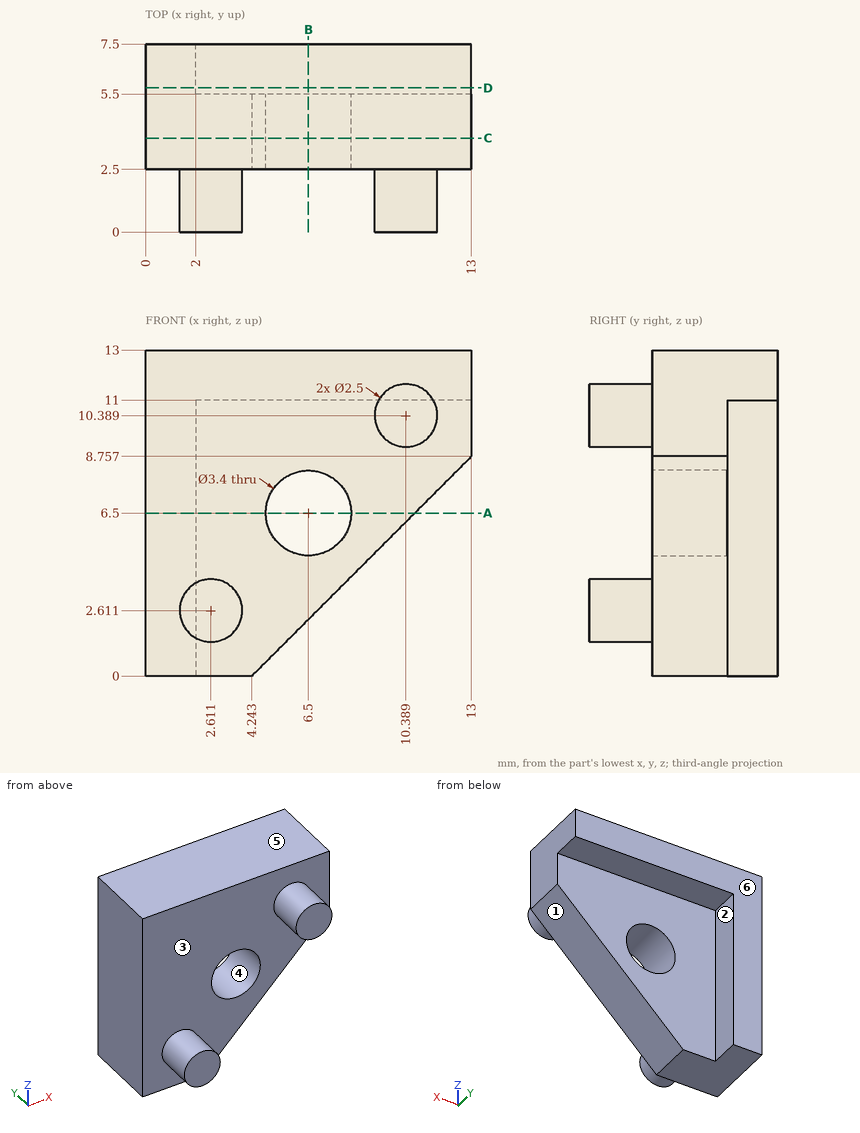
Design review of the part shown in the three views and the two pictorial views. Dimensions are in mm from the part's minimum x, y and z. A direction names the side the tool comes from. Give positions to 0.01 mm unless a question says otherwise; leave off trailing zeros. Loops run counter-clockwise (first coordinate to the right, second up) from the corner with the lowest first, then second, coordinate; pieces in that order, holes last. Notation, with made-up numbers: M 33.5,0.25 L 38.5,0.25 A17 ccw 38.5,22.25 Z; hole C -15.75,63.25 d9. An arc over 180 degrees is marked long. Answer as a JSON object with one key per item and string values. Group by question number.
Q1. Mouldability with a two-part tool opening along Z and no side actions: class the marked faces 4, 5 and 6 as +Z half, -Z half, draft (parallel to the pull), parting line (faces both ways), or undercut.
Q2. Add section B-B on x = 6.5. Give the boundary of the cut face in (y, z).
Q3. Tool access review of the marked faces 1, 2 and 3: name each direction out of +Z, -Z, +X, -X, +Y, -Y from which nothing blocks a thin tool from reaching the whole face with its end or side.
Q4. Add section C-C on y = 3.75. Give the boundary of the cut face in (x, z).
Q5. Insertion check: P1, Ø1, axis at x = 5.5, y = 7, coming from the -Z side; P2, Ø2, axis at x = 6.5, z = 9.5, coming from the -Y side; P3, Ø2, axis at x = 9.5, y = 6, coming from the -Z side. Each pin has a flat end and moves straight along its axis. Give the tip position at first contact, or say it passes through.
Q6. Add section A-A on z = 6.5. Give the boundary of the cut face in (x, y).
Q7. For probe 1 along X at (y, z) = (4.7, 6.5); probe 2 along Y at (x, z) = (3, 12); probe 3 along Y at (x, z) = (3.75, 7), list the stretches that pass through material, from the lowest coordinate up. Write a range as [from, to].
Q8. Add section D-D on y = 5.75. Give the boundary of the cut face in (x, z).
Checked values:
{
 "1": {"face 4": "undercut", "face 5": "+Z half", "face 6": "draft"},
 "2": {"outline": "M 2.5,2.26 L 5.5,2.26 L 5.5,4.8 L 2.5,4.8 Z; M 2.5,8.2 L 5.5,8.2 L 5.5,11 L 7.5,11 L 7.5,13 L 2.5,13 Z"},
 "3": {"face 1": "-Z, +X, +Y, -Y", "face 2": "-Z, +X, +Y", "face 3": "-Y"},
 "4": {"outline": "M 0,0 L 4.24,0 L 13,8.76 L 13,13 L 0,13 Z; hole C 6.5,6.5 d3.4"},
 "5": {"P1": "z = 11", "P2": "y = 2.5", "P3": "z = 4.39"},
 "6": {"outline": "M 0,2.5 L 4.8,2.5 L 4.8,5.5 L 2,5.5 L 2,7.5 L 0,7.5 Z; M 8.2,2.5 L 10.74,2.5 L 10.74,5.5 L 8.2,5.5 Z"},
 "7": {"probe 1": "[0, 4.8], [8.2, 10.74]", "probe 2": "[2.5, 7.5]", "probe 3": "[2.5, 5.5]"},
 "8": {"outline": "M 0,0 L 2,0 L 2,11 L 13,11 L 13,13 L 0,13 Z"}
}
